from build123d import *

# Parameters (mm, degrees)
F0_W     = 62
F0_H     = 15
F1_DEPTH = 3.4
F2_W     = 62
F2_H     = 0.7
F3_DEPTH = 2.5
F4_W     = 4.4
F4_H     = 1
F5_DEPTH = 1


with BuildPart() as f1:
    # F0 (on Top) → F1 (new body)
    with BuildSketch(Plane.XY):
        Rectangle(F0_W, F0_H)
    extrude(amount=F1_DEPTH)

    # F2 (on face) → F3 (join)
    with BuildSketch(Plane(origin=(0, 0, 0), x_dir=(1, 0, 0), z_dir=(0, 0, -1))):
        with Locations((0, -7.15)):
            Rectangle(F2_W, F2_H)
    extrude(amount=F3_DEPTH)

    # F4 (on face) → F5 (join)
    with BuildSketch(Plane.XZ.offset(7.5)):
        with Locations((-25.8, 1.7)):
            Rectangle(F4_W, F4_H)
        with Locations((-15.5, 1.7)):
            Rectangle(F4_W, F4_H)
        with Locations((-5.2, 1.7)):
            Rectangle(F4_W, F4_H)
        with Locations((5.1, 1.7)):
            Rectangle(F4_W, F4_H)
        with Locations((15.4, 1.7)):
            Rectangle(F4_W, F4_H)
        with Locations((25.7, 1.7)):
            Rectangle(F4_W, F4_H)
    extrude(amount=F5_DEPTH)


solid = f1.part
CAD build for the part. Positions are in the model's coordinates, mm. A direction names the side the tool comes from. Round coordinates to 2 decimals unless told otherwise and drop trailing zeros. Order: outer loops, then holes, each group sorted by start corner. A loop starts at its lowest first (then second) coordinate and runs counter-clockwise, first axis right, second up. Notation, with made-up numbers: (40, 20) -> (91, 20) arc R15 ccw to (91, 33) -> close; hole circle Ø6 at (25, -33.5). An arc over 180 degrees is marked (long way). Write item = value, one per line. Start each with the question number.
(1) Probe line 1 (Y direction, x = 8, z = 0.75); line 2 (Z direction, x = -25.5, y = 0); line 3 (Y direction, x = -7, z = -0.6). List the from-to ranges inside material, lowest first. Write a range as [from, to].
(2) Pin check, flat tips, straight feed: P1, Ø0.8, axis at y = -8, z = 1.5, coming from the +X side; P2, Ø0.5, axis at x = 15.5, y = -8, coming from the +Z side; P3, Ø8, axis at x = 4, y = 3.5, coming from the -Z side; P4, Ø0.8, axis at y = -8, z = 1.5, coming from the -X side. Stop position of each tip, or through.
(3) Cut at C-C, the plane z = -1.05. List the corners of the cut face in (x, y).
(4) Cut at D-D, the plane x = 9. List the corners of the cut face in (y, z).
(5) Cut at B-B, the plane y = -2.5. List the corners of the cut face in (x, z).
(6) Which spindle directions (+Z, -Z, +X, -X, +Y, -Y) get a long thin tool onto all of the face, cutting with end or side? Do faces 5 (the flat face through (-13.3, -8, 2)), 6 (the flat face through (-26, -8, 1.2)), 7 (the flat face through (5, -8, 2.2)). Say none if no direction does.
(7) Pull direction X, two halves, no side cores. Call faces 1 (the flat face through (0, -7.5, 2)), 2 (the flat face through (7.3, -8, 2)), 3 (the flat face through (-26, -8, 2.2)), 4 (the flat face through (-31, 0, 2)): released by +X, released by -X, zero draft, split by the parting line, or undercut.
(8) Cut at A-A, the plane x = -26. List the corners of the cut face in (y, z).
Model answer:
q1.line_1 = [-7.5, 7.5]
q1.line_2 = [0, 3.4]
q1.line_3 = [6.8, 7.5]
q2.P1 = 27.9
q2.P2 = 2.2
q2.P3 = -2.5
q2.P4 = -28
q3.outline = (-31, 6.8) -> (31, 6.8) -> (31, 7.5) -> (-31, 7.5) -> close
q4.outline = (-7.5, 0) -> (6.8, 0) -> (6.8, -2.5) -> (7.5, -2.5) -> (7.5, 3.4) -> (-7.5, 3.4) -> close
q5.outline = (-31, 0) -> (31, 0) -> (31, 3.4) -> (-31, 3.4) -> close
q6.face_5 = +Z, -Z, -Y
q6.face_6 = -Z, +X, -X, -Y
q6.face_7 = +Z, +X, -X, -Y
q7.face_1 = undercut
q7.face_2 = undercut
q7.face_3 = zero draft
q7.face_4 = released by -X
q8.outline = (-8.5, 1.2) -> (-7.5, 1.2) -> (-7.5, 0) -> (6.8, 0) -> (6.8, -2.5) -> (7.5, -2.5) -> (7.5, 3.4) -> (-7.5, 3.4) -> (-7.5, 2.2) -> (-8.5, 2.2) -> close
